Check sheet for the modelled part. Datum: model origin and axes. Units: mm. A direction names the side the tool comes from. Round coordinates to 2 decimals unless told otherwise and drop trailing zeros. Write each loop counter-clockwise with the first axis right and the second up, starting at its lowest first coordinate (ties: lowest second). Pieces come first, ordered by that corner, then holes.
Item 1: Material ranges on line 1 (X direction, y = 3, z = 109.5); line 2 (X direction, y = 44.5, z = 34.5); line 3 (Z direction, x = -1, y = 49), recorded low to high.
Item 2: Cross-section at A-A on z = 94. Enter the section's corners in (x, y), plus the area to 3 significant figures.
Item 3: Cross-section at B-B on z = 255. Enter the section's corners in (x, y), plus the area to 3 significant figures.
Item 4: Go/stop test with flat-tipped pins: pin 1 Ø1 at (x, z) = (14, 60) entering from +Y; pin 2 Ø6 at (x, y) = (23.5, 3) entering from +Z; pin 3 Ø8 at (y, z) = (-1.5, 352.5) entering from +X. Record where each tip stops, or that it passes through.
Item 5: Tool access check on faces 1 (the cylindrical face through (-19.8, 18.2, 274.9)), 2 (the flat face through (0, 22, 284)), 3 (the flat face through (0, -22, 284)). Record the directions out of +Z, -Z, +X, -X, +Y, -Y that give a thin tool (end or side, any length) a straight path to the whole face; none if there is none.
from build123d import *

# Parameters (mm, degrees)
F0_R       = 65
F1_DEPTH   = 200
F2_R       = 65
F3_DEPTH   = 66
F3_TAPER   = 30
F4_R       = 26.8948822335
F5_DEPTH   = 18
F6_W       = 38.8136626348
F6_H       = 37.2402786548
F7_DEPTH   = 26.9
F7_TAPER   = 15
F7_FACE_W  = 24.397996082
F7_FACE_H  = 22.824612102
F8_DEPTH   = 28.7
F8_TAPER   = 10
F10_DEPTH  = 126.2
F11_R      = 6.3517217046
F10_FACE_R = 6.3517217046
F12_DEPTH  = 10
F12_TAPER  = 30


with BuildPart() as f1:
    # F0 (on Top) → F1 (new body)
    with BuildSketch(Plane.XY):
        Circle(F0_R)
    extrude(amount=F1_DEPTH)

    # F2 (on face) → F3 (join)
    with BuildSketch(Plane.XY.offset(200)):
        Circle(F2_R)
    extrude(amount=F3_DEPTH, taper=F3_TAPER)

    # F4 (on face) → F5 (join)
    with BuildSketch(Plane.XY.offset(266)):
        Circle(F4_R)
    extrude(amount=F5_DEPTH)

    # F6 (on face) → F7 (join)
    with BuildSketch(Plane.XY.offset(284)):
        Rectangle(F6_W, F6_H)
    extrude(amount=F7_DEPTH, taper=F7_TAPER)

    # F7_face (on face) → F8 (join)
    with BuildSketch(Plane.XY.offset(310.9)):
        Rectangle(F7_FACE_W, F7_FACE_H)
    extrude(amount=F8_DEPTH, taper=F8_TAPER)

    # F9 (on face) → F10 (join)
    with BuildSketch(Plane.XY.offset(339.6)):
        with BuildLine():
            ThreePointArc((0, -6.3517217046), (4.4913454896, -4.4913454896), (6.3517217046, 0))
            ThreePointArc((6.3517217046, 0), (4.4913454896, 4.4913454896), (0, 6.3517217046))
            ThreePointArc((0, 6.3517217046), (-6.3517217046, 0), (0, -6.3517217046))
        make_face()
    extrude(amount=F10_DEPTH)

    # F11 (on face) + F10_face (on face) → F12 (join)
    with BuildSketch(Plane.XY.offset(465.8)):
        Circle(F11_R)
    with BuildSketch(Plane.XY.offset(465.8)):
        Circle(F10_FACE_R)
    extrude(amount=F12_DEPTH, taper=F12_TAPER)


solid = f1.part
Response values:
1. line 1: x = -64.93 to 64.93
1. line 2: x = -47.38 to 47.38
1. line 3: z = 0 to 227.7
2. outline: circle Ø130 at (0, 0)
2. area: 13,300 mm2
3. outline: circle Ø66.49 at (0, 0)
3. area: 3,470 mm2
4. pin 1: stops at y = 63.58
4. pin 2: stops at z = 284
4. pin 3: stops at x = 6.35
5. face 1: +Z
5. face 2: +Z, +X, -X, +Y
5. face 3: +Z, +X, -X, -Y
